```python
from build123d import *

# Parameters (mm, degrees)
SKETCH2_R          = 6.7183
CUT_EXTRUDE1_DEPTH = 56.211877571


with BuildPart() as part:
    # Sketch1 → Revolve1 (revolve)
    with BuildSketch(Plane.XY):
        with BuildLine():
            Line((-6.1595, 0), (-6.1595, 1.5875))
            ThreePointArc((-6.1595, 1.5875), (-7.435608029, 6.35), (-10.922, 9.836391971))
            Line((-10.922, 9.836391971), (-26.5811, 18.877177571))
            Line((-26.5811, 18.877177571), (-32.4739, 18.877177571))
            Line((-32.4739, 18.877177571), (-32.4739, -0.503022429))
            Line((-32.4739, -0.503022429), (-25.4, -0.503022429))
            Line((-25.4, -0.503022429), (-25.4, -36.3347))
            Line((-25.4, -36.3347), (-15.895353522, -36.3347))
            Line((-15.895353522, -36.3347), (-6.1595, 0))
        make_face()
    revolve(axis=Axis((0, 0, 0), (0, 1, 0)))

    # Sketch2 → Cut-Extrude1 (cut, through all)
    with BuildSketch(Plane(origin=(0, 18.877177571, 0), x_dir=(1, 0, 0), z_dir=(0, 1, 0))):
        Circle(SKETCH2_R)
    extrude(amount=-CUT_EXTRUDE1_DEPTH, mode=Mode.SUBTRACT)


solid = part.part
```
The model under review builds one solid part; all positions refer to its coordinate system, in mm. A direction names the side the tool comes from. Give positions to 0.01 mm unless a question says otherwise; leave off trailing zeros. Write each loop counter-clockwise with the first axis right and the second up, starting at its lowest first coordinate (ties: lowest second). Pieces come first, ordered by that corner, then holes. Notation, with made-up numbers: (68, 14) -> (114, 14) arc R17 cw to (114, 19) -> close; hole circle Ø9 at (-26, 83). An arc over 180 degrees is marked (long way). Answer in a Markdown table with one row per item.
1) Tool access review of faces 1 (the conical face through (-5.49, 10.4, -10.56)), 2 (the flat face through (19.4, -0.503, -16.7)): name each direction out of +Z, -Z, +X, -X, +Y, -Y from which nothing blocks a thin tool from reaching the whole face with its end or side.
Worked answers:
| item | result |
|---|---|
| face 1 | +Y |
| face 2 | -Y |
2) Mouldability with a two-part tool opening along Z and no side actions: class faces 3 (the flat face through (-27, 18.877, 0)), 4 (the conical face through (2.216, -15.165, -9.98)), 5 (the cylindrical face through (5.506, -18.67, -24.796)) as +Z half, -Z half, draft (parallel to the pull), parting line (faces both ways), or undercut.
Worked answers:
| item | result |
|---|---|
| face 3 | draft |
| face 4 | undercut |
| face 5 | parting line |
3) Add section C-C on y = -22. State the section outline as (x, z) points, plus the area to 3 significant figures.
Worked answers:
| item | result |
|---|---|
| outline | circle Ø50.8 at (0, 0); hole circle Ø24.11 at (0, 0) |
| area | 1,570 mm² |
4) Clearance check with flat-ended pins moving along their axes: P1, Ø3, axis at y = -9.5, z = 25, coming from the +X side; P2, Ø5, axis at x = -13.5, z = 10, coming from the +Y side; P3, Ø4, axis at x = -8, z = 7.5, coming from the +Y side. State where each tip first meets the part, or that it passes through.
Worked answers:
| item | result |
|---|---|
| P1 | x = 9.64 |
| P2 | y = 14.67 |
| P3 | y = 11.02 |
5) Add section D-D on y = 15.5. State the section outline as (x, z) points, plus the area to 3 significant figures.
Worked answers:
| item | result |
|---|---|
| outline | circle Ø64.95 at (0, 0); hole circle Ø41.46 at (0, 0) |
| area | 1,960 mm² |
6) For L1, parallel to Z at x = 0, y = 1.5; L2, parallel to Y at x = 22.5, z = 17; L3, parallel to X at y = 9, z = -2.5, list the stretches that pass through material, from the lowest coordinate up. Write a range as [from, to].
Worked answers:
| item | result |
|---|---|
| L1 | [-32.47, -6.72], [6.72, 32.47] |
| L2 | [-0.5, 18.88] |
| L3 | [-32.38, -9.38], [9.38, 32.38] |
